from build123d import *

# Parameters (mm, degrees)
EXTRUDE_1_DEPTH = 440


with BuildPart() as part:
    # 草圖1 → 填料-伸長1 (new body)
    with BuildSketch(Plane.XY):
        Polygon((0, 0), (17.69379362, -17.661530719), (0.032262901, -35.355324339), (-17.661530719, -17.69379362), align=None)
        Polygon((0.001935774, -2.12131946), (-15.540211259, -17.691857846), (0.030327127, -33.234004879), (15.57247416, -17.663466493), align=None, mode=Mode.SUBTRACT)
    extrude(amount=EXTRUDE_1_DEPTH)


solid = part.part
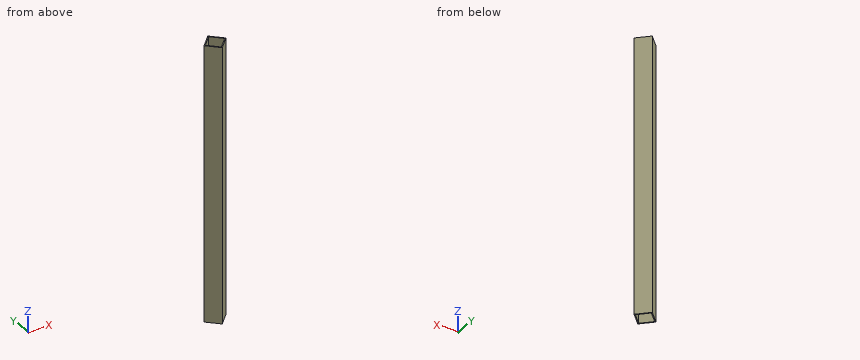
The model under review builds one solid part; all positions refer to its coordinate system, in mm. Round coordinates to 2 decimals unless told otherwise and drop trailing zeros. Loops run counter-clockwise (first coordinate to the right, second up) from the corner with the lowest first, then second, coordinate; pieces in that order, holes last. Notation, with made-up numbers: (-6.5, -13) - (28.5, -13) arc R11 ccw to (28.5, -1) - close; hole circle Ø10 at (56.25, 64.5). An arc over 180 degrees is marked (long way). Use CSV: the item, a comma, the result in double quotes.
(1) Take a section at A-A, the plane z = 370.5. Give the boundary of the cut face in (x, y), plus the area to 3 significant figures.
Working result:
outline,"(-17.66, -17.69) - (0.03, -35.36) - (17.69, -17.66) - (0, 0) - close; hole (-15.54, -17.69) - (0.03, -33.23) - (15.57, -17.66) - (0, -2.12) - close"
area,"141 mm^2"
(2) For line 1 (Y direction, x = -3, z = 248); line 2 (X direction, y = -22, z = 232.5); line 3 (Y direction, x = -1.5, z = 96.5), list the stretches that pass through material, from the lowest coordinate up.
Working result:
line 1,"y = -32.33 to -30.21, -5.13 to -3.01"
line 2,"x = -13.35 to -11.22, 11.24 to 13.36"
line 3,"y = -33.83 to -31.71, -3.63 to -1.5"
(3) Clearance check with flat-ended pins moving along their axes: P1, Ø1, axis at y = -29, z = 71, coming from the +X side; P2, Ø5, axis at x = 0, z = 249, coming from the +Y side; P3, Ø12, axis at x = 7, z = 228, coming from the +Y side. State where each tip first meets the part, or that it passes through.
Working result:
P1,"stops at x = 6.88"
P2,"stops at y = 0"
P3,"stops at y = -1"
(4) Take a section at C-C, the plane x = -9. Give the boundary of the cut face in (y, z), plus the area to 3 significant figures.
Working result:
outline,"(-26.34, 0) - (-24.22, 0) - (-24.22, 440) - (-26.34, 440) - close; (-11.14, 0) - (-9.02, 0) - (-9.02, 440) - (-11.14, 440) - close"
area,"1,870 mm^2"
(5) Take a section at B-B, the plane y = -6. Give the boundary of the cut face in (x, z).
Working result:
outline,"(-5.99, 0) - (-3.87, 0) - (-3.87, 440) - (-5.99, 440) - close; (3.89, 0) - (6.01, 0) - (6.01, 440) - (3.89, 440) - close"
